```python
from build123d import *

# Parameters (mm, degrees)
F0_W         = 100
F0_H         = 37.7952754252
F1_DEPTH     = 200
F2_W         = 80
F2_H         = 30
F3_DEPTH     = 5
F4_T4_DEPTH  = 55.4
F4_T9_DEPTH  = 105.4
F4_T14_DEPTH = 55.4
F4_T19_DEPTH = 105.4
F5_W         = 100
F5_H         = 155.959841609
F6_DEPTH     = 3
F7_W         = 18.5192480683
F7_H         = 2.9272809625
F7_W_2       = 4.0360428393
F7_W_3       = 4.3243318796
F7_W_4       = 4.4076992199
F7_W_5       = 4.324331414
F7_W_6       = 4.9009080976
F7_W_7       = 4.6126190573
F7_W_8       = 16.3274921477
F8_DEPTH     = 3
F9_W         = 3.4559369087
F9_H         = 2.9272809625
F9_W_2       = 3.5711340606
F9_W_3       = 3.2255388796
F10_DEPTH    = 3
F11_R        = 5.08
F12_R        = 1


# Not quite as in the source:
# - a fillet or chamfer that OpenCascade refuses, or shapes differently, is made with other operations: its cross-section is extruded or revolved along the edge and cut away or added


with BuildPart() as f1:
    # F0 (on Front) → F1 (new body)
    with BuildSketch(Plane.XZ):
        with Locations((-0.3143809736, 22.1638707444)):
            Rectangle(F0_W, F0_H)
    extrude(amount=F1_DEPTH)

    # F2 (on face) → F3 (join)
    with BuildSketch(Plane.XY.offset(41.061508457)):
        with Locations((-0.3143809736, -24.2907730862)):
            Rectangle(F2_W, F2_H)
    extrude(amount=F3_DEPTH)

    # F4: fillet of radius 5.08 on 4 edges, made by hand


with BuildPart() as f4_tool2:
    # F4_s3 → F4_t4 (new body)
    with BuildSketch(Plane.XZ.offset(51.9907730862)):
        with BuildLine():
            ThreePointArc((39.6856190264, 40.981508457), (38.1977214749, 44.5736109055), (34.6056190264, 46.061508457))
            Line((34.6056190264, 46.061508457), (39.6856190264, 46.061508457))
            Line((39.6856190264, 46.061508457), (39.6856190264, 40.981508457))
        make_face()
    extrude(amount=-F4_T4_DEPTH)

    split(bisect_by=Plane.XY.offset(41.061508457), keep=Keep.TOP)


with BuildPart() as f1_1:
    add(f1.part)

    # F4_t1: cut F4_tool2
    add(f4_tool2.part, mode=Mode.SUBTRACT)


with BuildPart() as f4_tool7:
    # F4_s8 → F4_t9 (new body)
    with BuildSketch(Plane.YZ.offset(52.3856190264)):
        with BuildLine():
            ThreePointArc((-9.2907730862, 40.981508457), (-10.7786706378, 44.5736109055), (-14.3707730862, 46.061508457))
            Line((-14.3707730862, 46.061508457), (-9.2907730862, 46.061508457))
            Line((-9.2907730862, 46.061508457), (-9.2907730862, 40.981508457))
        make_face()
    extrude(amount=-F4_T9_DEPTH)

    split(bisect_by=Plane.XY.offset(41.061508457), keep=Keep.TOP)


with BuildPart() as f1_2:
    add(f1_1.part)

    # F4_t6: cut F4_tool7
    add(f4_tool7.part, mode=Mode.SUBTRACT)


with BuildPart() as f4_tool12:
    # F4_s13 → F4_t14 (new body)
    with BuildSketch(Plane.XZ.offset(-3.4092269138)):
        with BuildLine():
            ThreePointArc((-40.3143809736, 40.981508457), (-38.826483422, 44.5736109055), (-35.2343809736, 46.061508457))
            Line((-35.2343809736, 46.061508457), (-40.3143809736, 46.061508457))
            Line((-40.3143809736, 46.061508457), (-40.3143809736, 40.981508457))
        make_face()
    extrude(amount=F4_T14_DEPTH)

    split(bisect_by=Plane.XY.offset(41.061508457), keep=Keep.TOP)


with BuildPart() as f1_3:
    add(f1_2.part)

    # F4_t11: cut F4_tool12
    add(f4_tool12.part, mode=Mode.SUBTRACT)


with BuildPart() as f4_tool17:
    # F4_s18 → F4_t19 (new body)
    with BuildSketch(Plane.YZ.offset(-53.0143809736)):
        with BuildLine():
            ThreePointArc((-39.2907730862, 40.981508457), (-37.8028755347, 44.5736109055), (-34.2107730862, 46.061508457))
            Line((-34.2107730862, 46.061508457), (-39.2907730862, 46.061508457))
            Line((-39.2907730862, 46.061508457), (-39.2907730862, 40.981508457))
        make_face()
    extrude(amount=F4_T19_DEPTH)

    split(bisect_by=Plane.XY.offset(41.061508457), keep=Keep.TOP)


with BuildPart() as f1_4:
    add(f1_3.part)

    # F4_t16: cut F4_tool17
    add(f4_tool17.part, mode=Mode.SUBTRACT)

    # F5 (on face) → F6 (join)
    with BuildSketch(Plane.XY.offset(41.061508457)):
        with Locations((-0.3143809736, -122.0200791955)):
            Rectangle(F5_W, F5_H)
    extrude(amount=F6_DEPTH)

    # F7 (on face) → F8 (join)
    with BuildSketch(Plane.XY.offset(41.061508457)):
        with Locations((-41.0547569394, -42.5765179098)):
            Rectangle(F7_W, F7_H)
        with Locations((-26.0293576866, -42.5765179098)):
            Rectangle(F7_W_2, F7_H)
        with Locations((-17.9572720081, -42.5765179098)):
            Rectangle(F7_W_2, F7_H)
        with Locations((-10.31761989, -42.5765179098)):
            Rectangle(F7_W_3, F7_H)
        with Locations((-2.2038496099, -42.5765179098)):
            Rectangle(F7_W_4, F7_H)
        with Locations((5.2499750163, -42.5765179098)):
            Rectangle(F7_W_5, F7_H)
        with Locations((12.7454819158, -42.5765179098)):
            Rectangle(F7_W_3, F7_H)
        with Locations((20.817569457, -42.5765179098)):
            Rectangle(F7_W_6, F7_H)
        with Locations((28.4572215751, -42.5765179098)):
            Rectangle(F7_W_7, F7_H)
        with Locations((41.5218729526, -42.5765179098)):
            Rectangle(F7_W_8, F7_H)
    extrude(amount=F8_DEPTH)

    # F9 (on face) → F10 (cut)
    with BuildSketch(Plane.XY.offset(44.061508457)):
        with Locations((-37.5542342663, -42.5765179098)):
            Rectangle(F9_W, F9_H)
        with Locations((-44.8692981154, -42.5765179098)):
            Rectangle(F9_W_2, F9_H)
        with Locations((38.4763423353, -42.5765179098)):
            Rectangle(F9_W_3, F9_H)
        with Locations((44.8122248054, -42.5765179098)):
            Rectangle(F9_W, F9_H)
    extrude(amount=-F10_DEPTH, mode=Mode.SUBTRACT)

    # F11
    f11_edges = [f1_4.edges().sort_by_distance(p)[0] for p in [
        (-0.314381, -200, 44.061508),
    ]]
    fillet(f11_edges, radius=F11_R)

    # F12
    f12_edges = [f1_4.edges().sort_by_distance(p)[0] for p in [
        (49.685619, -20.556439, 41.061508),
        (-0.314381, 0, 41.061508),
        (-50.314381, -20.556439, 41.061508),
        (-50.314381, -118.016439, 44.061508),
        (49.685619, -118.016439, 44.061508),
    ]]
    fillet(f12_edges, radius=F12_R)


solid = f1_4.part
```
Part model, mm, in its own coordinate system. A direction names the side the tool comes from. Round coordinates to 2 decimals unless told otherwise and drop trailing zeros. Loops run counter-clockwise (first coordinate to the right, second up) from the corner with the lowest first, then second, coordinate; pieces in that order, holes last. Notation, with made-up numbers: (6, 52.25) -> (58, 52.25) arc R22 ccw to (58, 78.25) -> close; hole circle Ø5 at (57.25, 10.25). An arc over 180 degrees is marked (long way). Use CSV: the item, a comma, the result in double quotes. Start each with the question number.
1) Wall check: L1, parallel to Z at x = -19.5, y = -112.5; L2, parallel to Z at x = 46.5, y = -32; L3, parallel to X at y = -15.5, z = 43.5. Give the ranges that are in metal, low to high. Write a range as [from, to].
2) Pull direction Y, two halves, no side cores. Call faces 4 (the cylindrical face through (0.246, -10.768, 44.563)), 5 (the cylindrical face through (-38.8, -24.1, 44.6)), 6 (the flat face through (-1, -200, 21)), 7 (the cylindrical face through (-0.874, -37.814, 44.563)): +Y half, -Y half, draft (parallel to the pull), parting line (faces both ways), or undercut.
3) Cut at A-A, the plane y = -66. Write the cut outline in (x, z).
4) Drop flat-ended pins along their axis: P1, Ø1.5, axis at x = 45.5, z = 43, coming from the +Y side; P2, Ø0.9, axis at x = -34.5, z = 42.5, coming from the +Y side; P3, Ø12, axis at x = -8, z = 40.5, coming from the -Y side; P4, Ø8, axis at x = 22, y = -151.5, coming from the +Z side. Give the stop position or say it passes through.
5) Which spindle directions (+Z, -Z, +X, -X, +Y, -Y) get a long thin tool onto all of the face, cutting with end or side? Do faces 1 (the flat face through (-1, 0, 22)), 2 (the cylindrical face through (38.21, -24.5, 44.56)), 3 (the flat face through (-1, -117, 44.062)). Say none if no direction does.
Determined:
1,L1,"z = [3.27, 44.06]"
1,L2,"z = [3.27, 41.06]"
1,L3,"x = [-39.65, 39.02]"
2,face 4,"+Y half"
2,face 5,"draft"
2,face 6,"-Y half"
2,face 7,"undercut"
3,outline,"(-50.31, 3.27) -> (49.69, 3.27) -> (49.69, 43.06) arc R1 ccw to (48.69, 44.06) -> (-49.31, 44.06) arc R1 ccw to (-50.31, 43.06) -> close"
4,P1,"stops at y = -44.04"
4,P2,"stops at y = -9.4"
4,P3,"stops at y = -200"
4,P4,"stops at z = 44.06"
5,face 1,"+Z, -Z, +X, -X, +Y"
5,face 2,"+Z, +X, +Y"
5,face 3,"+Z, +X, -X, -Y"
